Build history of the part. All positions in model axes, mm. A direction names the side the tool comes from. Give positions to 0.01 mm unless a question says otherwise; leave off trailing zeros. Write each loop counter-clockwise with the first axis right and the second up, starting at its lowest first coordinate (ties: lowest second). Pieces come first, ordered by that corner, then holes.
from build123d import *

# Parameters (mm, degrees)
SKETCH1_W           = 32.5
SKETCH1_H           = 6
SKETCH1_R           = 1.75
BOSS_EXTRUDE1_DEPTH = 3
SKETCH2_W           = 21.36
SKETCH2_H           = 12
BOSS_EXTRUDE2_DEPTH = 3
SKETCH3_W           = 35
SKETCH3_H           = 5
BOSS_EXTRUDE3_DEPTH = 3
SKETCH4_W           = 6
SKETCH4_H           = 5
BOSS_EXTRUDE4_DEPTH = 12.5
SKETCH5_W           = 35
SKETCH5_H           = 15
BOSS_EXTRUDE5_DEPTH = 7.8
CHAMFER1_SIZE       = 2.5
SKETCH6_R           = 1.75
CUT_EXTRUDE1_DEPTH  = 35.22718218
BOSS_EXTRUDE6_DEPTH = 1
SKETCH8_W           = 32.5
SKETCH8_H           = 1
BOSS_EXTRUDE7_DEPTH = 27.5
CUT_EXTRUDE2_DEPTH  = 33.5
CUT_EXTRUDE3_DEPTH  = 52.775500963


with BuildPart() as part:
    # Sketch1 → Boss-Extrude1 (new body)
    with BuildSketch(Plane(origin=(0, 0, 0), x_dir=(1, 0, 0), z_dir=(0, 1, 0))):
        Rectangle(SKETCH1_W, SKETCH1_H)
        with Locations(Location((-12.7, 0, 0), (0, 0, 270))):
            Circle(SKETCH1_R, mode=Mode.SUBTRACT)
        with Locations(Location((12.7, 0, 0), (0, 0, 90))):
            Circle(SKETCH1_R, mode=Mode.SUBTRACT)
    extrude(amount=BOSS_EXTRUDE1_DEPTH)

    # Sketch2 → Boss-Extrude2 (add)
    with BuildSketch(Plane.XZ):
        with Locations((0, -9)):
            Rectangle(SKETCH2_W, SKETCH2_H)
    extrude(amount=-BOSS_EXTRUDE2_DEPTH)

    # Sketch3 → Boss-Extrude3 (add)
    with BuildSketch(Plane.XZ):
        with Locations((0, -12.5)):
            Rectangle(SKETCH3_W, SKETCH3_H)
    extrude(amount=-BOSS_EXTRUDE3_DEPTH)

    # Sketch4 → Boss-Extrude4 (add)
    with BuildSketch(Plane(origin=(0, 3, 0), x_dir=(1, 0, 0), z_dir=(0, 1, 0))):
        with Locations((-14.5, 12.5)):
            Rectangle(SKETCH4_W, SKETCH4_H)
        with Locations((14.5, 12.5)):
            Rectangle(SKETCH4_W, SKETCH4_H)
    extrude(amount=BOSS_EXTRUDE4_DEPTH)

    # Sketch5 → Boss-Extrude5 (add)
    with BuildSketch(Plane(origin=(0, 15.5, 0), x_dir=(1, 0, 0), z_dir=(0, 1, 0))):
        with Locations((0, 17.5)):
            Rectangle(SKETCH5_W, SKETCH5_H)
    extrude(amount=BOSS_EXTRUDE5_DEPTH)

    # Chamfer1
    chamfer1_edges = [part.edges().sort_by_distance(p)[0] for p in [
        (0, 23.3, -10),
    ]]
    chamfer(chamfer1_edges, length=CHAMFER1_SIZE)

    # Sketch6 → Cut-Extrude1 (cut, through all)
    with BuildSketch(Plane.XZ.offset(-15.5)):
        with Locations(Location((-12.5, -20, 0), (0, 0, 270))):
            Circle(SKETCH6_R)
        with Locations(Location((12.5, -20, 0), (0, 0, 90))):
            Circle(SKETCH6_R)
    extrude(amount=-CUT_EXTRUDE1_DEPTH, mode=Mode.SUBTRACT)

    # Sketch7 → Boss-Extrude6 (add)
    with BuildSketch(Plane.ZY.offset(16.25)):
        Polygon((-3, 2), (-3, 18.8), (30.5, 2), align=None)
    boss_extrude6 = extrude(amount=BOSS_EXTRUDE6_DEPTH)

    # Mirror1: Boss-Extrude6 across plane
    add(boss_extrude6.mirror(Plane(origin=(0, 0, 0), x_dir=(0, 0, 1), z_dir=(1, 0, 0))))

    # Sketch8 → Boss-Extrude7 (add)
    with BuildSketch(Plane.XY.offset(3)):
        with Locations((0, 2.5)):
            Rectangle(SKETCH8_W, SKETCH8_H)
    extrude(amount=BOSS_EXTRUDE7_DEPTH)

    # Sketch9 → Cut-Extrude2 (cut)
    with BuildSketch(Plane(origin=(16.25, 0, 0), x_dir=(0, 0, -1), z_dir=(1, 0, 0))):
        Polygon((-30.5, 2), (-28.505952381, 3), (-30.5, 3), align=None)
    extrude(amount=-CUT_EXTRUDE2_DEPTH, mode=Mode.SUBTRACT)

    # Sketch10 → Cut-Extrude3 (cut, through all)
    with BuildSketch(Plane.ZY.offset(17.25)):
        Polygon((-3, 15), (4.577380952, 15), (-3, 18.8), align=None)
    extrude(amount=-CUT_EXTRUDE3_DEPTH, mode=Mode.SUBTRACT)


solid = part.part
1. Saw through at A-A on z = 0. Give the cut face in (x, y).
2. Saw through at B-B on x = 5.5. Give the cut face in (y, z), plus the area to 3 significant figures.
3. Drill centre lines: line 1 along X through (y, z) = (18, -20); line 2 along X through (y, z) = (2.25, 0); line 3 along Z through (x, y) = (12.7, 0.85). Where is each one in solid material? Low to high.
4. Saw through at C-C on y = 5.5. Give the cut face in (x, z), plus the area to 3 significant figures.
5. 3-axis set-ups, long thin cutter, end or side, ignore diameter. For faces 4 (the face through (0, 15.5, -18)), 5 (the face through (-16.25, 8, 9)), 6 (the face through (16.25, 1, 0)), 7 (the face through (-16.25, 1, 0)): which of +Z, -Z, +X, -X, +Y, -Y reach the whole face in a straight line?
6. Saw through at D-D on z = -20. Give the cut face in (x, y), plus the area to 3 significant figures.
7. Drop flat-ended pins along their axis: pin 1 (0.5 mm diameter, centred on x = 17, z = 1.5, fed in from +Y); pin 2 (0.6 mm diameter, centred on x = 8, y = 1, fed in from +Z); pin 3 (6 mm diameter, centred on y = 19.5, z = 7, fed in from -X); pin 4 (10.5 mm diameter, centred on y = 7, z = 8, fed in from -X). Give the stop position or say it passes through.
8. Mould opens along Z. For faces 1 (the face through (17.25, 7, 10)), 2 (the face through (-11.32, 19.35, -18.71)), 3 (the face through (0, 19, -25)) say: pulls with the +Z half, pulls with the -Z half, needs draft (parallel to the pull), parting line crosses it, or undercut.
Outcome:
1. outline: (-17.25, 2) - (-16.25, 2) - (-16.25, 0) - (-14.45, 0) - (-14.45, 3) - (-16.25, 3) - (-16.25, 15) - (-17.25, 15) - close; (-10.95, 0) - (10.95, 0) - (10.95, 3) - (-10.95, 3) - close; (14.45, 0) - (16.25, 0) - (16.25, 2) - (17.25, 2) - (17.25, 15) - (16.25, 15) - (16.25, 3) - (14.45, 3) - close
2. outline: (0, -15) - (3, -15) - (3, 28.51) - (2, 30.5) - (2, 3) - (0, 3) - close; (15.5, -25) - (23.3, -25) - (23.3, -12.5) - (20.8, -10) - (15.5, -10) - close
2. area: 194 mm2
3. line 1: x = -17.5 to -14.25, -10.75 to 10.75, 14.25 to 17.5
3. line 2: x = -17.25 to -14.45, -10.95 to 10.95, 14.45 to 17.25
3. line 3: z = -15 to -10, -3 to -1.75, 1.75 to 3
4. outline: (-17.5, -15) - (-11.5, -15) - (-11.5, -10) - (-17.5, -10) - close; (-17.25, -3) - (-16.25, -3) - (-16.25, 23.52) - (-17.25, 23.52) - close; (11.5, -15) - (17.5, -15) - (17.5, -10) - (11.5, -10) - close; (16.25, -3) - (17.25, -3) - (17.25, 23.52) - (16.25, 23.52) - close
4. area: 113 mm2
5. face 4: -Z
5. face 5: +Z, +Y
5. face 6: +Z, +X, -Y
5. face 7: +Z, -X, -Y
6. outline: (-17.5, 15.5) - (-14.25, 15.5) - (-14.25, 23.3) - (-17.5, 23.3) - close; (-10.75, 15.5) - (10.75, 15.5) - (10.75, 23.3) - (-10.75, 23.3) - close; (14.25, 15.5) - (17.5, 15.5) - (17.5, 23.3) - (14.25, 23.3) - close
6. area: 218 mm2
7. pin 1: stops at y = 15
7. pin 2: stops at z = 3
7. pin 3: passes through
7. pin 4: stops at x = -17.25
8. face 1: needs draft
8. face 2: undercut
8. face 3: pulls with the -Z half
